Model file for the job. Use its own axes, mm. A direction names the side the tool comes from. Coordinates: 2 decimals unless noted, no trailing zeros. Loops run counter-clockwise (first coordinate to the right, second up) from the corner with the lowest first, then second, coordinate; pieces in that order, holes last.
from build123d import *

# Parameters (mm, degrees)
F0_W      = 47.7012
F0_H      = 9.5758
F1_DEPTH  = 7.8232
F2_R      = 2.3876
F3_DEPTH  = 9.53232
F2_R_2    = 3.0048968535
F2_R_3    = 2.9922132855
F2_R_4    = 2.9972531663
F4_DEPTH  = 0.762
F5_R      = 2.9885913722
F5_R_2    = 3.0048968535
F5_R_3    = 2.9922132855
F5_R_4    = 2.9972531663
F5_R_5    = 2.9570387739
F6_DEPTH  = 25.4
F7_R      = 3.0048968535
F7_R_2    = 2.3876
F7_R_3    = 2.9922132855
F7_R_4    = 2.9972531663
F7_R_5    = 2.9885913722
F7_R_6    = 2.9570387739
F8_DEPTH  = 0.762
F9_R      = 2.4384
F9_R_2    = 1.6002
F10_DEPTH = 0.9398
F11_W     = 45.9232
F11_H     = 6.0452
F12_DEPTH = 2.794


with BuildPart() as f1:
    # F0 (on Front) → F1 (new body)
    with BuildSketch(Plane.XZ):
        with Locations((-0.3360249102, 0.7659190055)):
            Rectangle(F0_W, F0_H)
    extrude(amount=F1_DEPTH)

    # F2 (on Front) → F3 (cut)
    with BuildSketch(Plane.XZ):
        with Locations((15.0480590754, 1.8556544835)):
            Circle(F2_R)
        with BuildLine():
            Line((5.7234941433, 0), (8.8326681668, 3.624302958))
            ThreePointArc((8.8326681668, 3.624302958), (5.4659296761, 3.3667384908), (5.7234941433, 0))
        make_face()
        with BuildLine():
            ThreePointArc((5.7234941433, 0), (8.275302748, -0.3572223603), (9.6656811551, 1.812151479))
            ThreePointArc((9.6656811551, 1.812151479), (9.4474549944, 2.8093730719), (8.8326681668, 3.624302958))
            Line((8.8326681668, 3.624302958), (5.7234941433, 0))
        make_face()
        with BuildLine():
            Line((-2.2399391754, 0.0756290061), (0.8692348481, 3.6999319641))
            ThreePointArc((0.8692348481, 3.6999319641), (-2.4975036427, 3.4423674968), (-2.2399391754, 0.0756290061))
        make_face()
        with BuildLine():
            ThreePointArc((-2.2399391754, 0.0756290061), (0.3118694292, -0.2815933542), (1.7022478363, 1.8877804851))
            ThreePointArc((1.7022478363, 1.8877804851), (1.4840216756, 2.885002078), (0.8692348481, 3.6999319641))
            Line((0.8692348481, 3.6999319641), (-2.2399391754, 0.0756290061))
        make_face()
        with BuildLine():
            Line((-9.9647576041, 0), (-7.3799977582, 4.0151651995))
            ThreePointArc((-7.3799977582, 4.0151651995), (-10.6799602808, 3.2999625227), (-9.9647576041, 0))
        make_face()
        with BuildLine():
            ThreePointArc((-9.9647576041, 0), (-7.5289295065, -0.0884040491), (-6.2847776811, 2.0075825997))
            ThreePointArc((-6.2847776811, 2.0075825997), (-6.5763910323, 3.1510307743), (-7.3799977582, 4.0151651995))
            Line((-7.3799977582, 4.0151651995), (-9.9647576041, 0))
        make_face()
        with BuildLine():
            Line((-17.9671654597, 0), (-15.2041278281, 3.8946319578))
            ThreePointArc((-15.2041278281, 3.8946319578), (-18.5329626228, 3.3288347947), (-17.9671654597, 0))
        make_face()
        with BuildLine():
            ThreePointArc((-17.9671654597, 0), (-15.4897179429, -0.1739039631), (-14.1980466439, 1.9473159789))
            ThreePointArc((-14.1980466439, 1.9473159789), (-14.4644267019, 3.0432446799), (-15.2041278281, 3.8946319578))
            Line((-15.2041278281, 3.8946319578), (-17.9671654597, 0))
        make_face()
    extrude(amount=F3_DEPTH, mode=Mode.SUBTRACT)

    # F2 (on Front) → F4 (cut)
    with BuildSketch(Plane.XZ):
        with BuildLine():
            ThreePointArc((-16.5209776811, 4.9036475293), (-16.5856466439, 4.9043547528), (-16.6503156067, 4.9036475293))
            Line((-16.6503156067, 4.9036475293), (-16.5209776811, 4.9036475293))
        make_face()
        with BuildLine():
            ThreePointArc((-5.6837863089, 2.0075825997), (-6.8384723861, 4.3673431298), (-9.41027084, 4.9036475293))
            ThreePointArc((-9.41027084, 4.9036475293), (-10.5062829761, -0.3521779303), (-5.6837863089, 2.0075825997))
        make_face()
        with BuildLine():
            ThreePointArc((-7.3799977582, 4.0151651995), (-6.5763910323, 3.1510307743), (-6.2847776811, 2.0075825997))
            ThreePointArc((-6.2847776811, 2.0075825997), (-7.5289295065, -0.0884040491), (-9.9647576041, 0))
            ThreePointArc((-9.9647576041, 0), (-10.6799602808, 3.2999625227), (-7.3799977582, 4.0151651995))
        make_face(mode=Mode.SUBTRACT)
        with BuildLine():
            Line((-16.5209776811, 4.9036475293), (-16.6503156067, 4.9036475293))
            ThreePointArc((-16.6503156067, 4.9036475293), (-18.5630084962, 4.1459788488), (-19.5185854293, 2.3240763694))
            ThreePointArc((-19.5185854293, 2.3240763694), (-18.8162584098, 0.0060665204), (-16.6174061088, -1.0095522371))
            ThreePointArc((-16.6174061088, -1.0095522371), (-14.5059634539, -0.1548248679), (-13.6286078699, 1.9473159789))
            ThreePointArc((-13.6286078699, 1.9473159789), (-14.4719642007, 4.0152678256), (-16.5209776811, 4.9036475293))
        make_face()
        with BuildLine():
            ThreePointArc((-15.2041278281, 3.8946319578), (-14.4644267019, 3.0432446799), (-14.1980466439, 1.9473159789))
            ThreePointArc((-14.1980466439, 1.9473159789), (-15.4897179429, -0.1739039631), (-17.9671654597, 0))
            ThreePointArc((-17.9671654597, 0), (-18.5329626228, 3.3288347947), (-15.2041278281, 3.8946319578))
        make_face(mode=Mode.SUBTRACT)
        with Locations((-0.6853521637, 1.8877804851)):
            Circle(F2_R_2)
        with BuildLine():
            ThreePointArc((0.8692348481, 3.6999319641), (1.4840216756, 2.885002078), (1.7022478363, 1.8877804851))
            ThreePointArc((1.7022478363, 1.8877804851), (0.3118694292, -0.2815933542), (-2.2399391754, 0.0756290061))
            ThreePointArc((-2.2399391754, 0.0756290061), (-2.4975036427, 3.4423674968), (0.8692348481, 3.6999319641))
        make_face(mode=Mode.SUBTRACT)
        with Locations((7.2780811551, 1.812151479)):
            Circle(F2_R_3)
        with BuildLine():
            ThreePointArc((8.8326681668, 3.624302958), (9.4474549944, 2.8093730719), (9.6656811551, 1.812151479))
            ThreePointArc((9.6656811551, 1.812151479), (8.275302748, -0.3572223603), (5.7234941433, 0))
            ThreePointArc((5.7234941433, 0), (5.4659296761, 3.3667384908), (8.8326681668, 3.624302958))
        make_face(mode=Mode.SUBTRACT)
        with Locations((15.0480590754, 1.8556544835)):
            Circle(F2_R_4)
        with Locations((15.0480590754, 1.8556544835)):
            Circle(F2_R, mode=Mode.SUBTRACT)
    extrude(amount=F4_DEPTH, mode=Mode.SUBTRACT)

    # F5 (on Front) → F6 (cut)
    with BuildSketch(Plane.XZ):
        with Locations((-8.6723776811, 2.0075825997)):
            Circle(F5_R)
        with Locations((-0.6853521637, 1.8877804851)):
            Circle(F5_R_2)
        with Locations((7.2780811551, 1.812151479)):
            Circle(F5_R_3)
        with Locations((15.0480590754, 1.8556544835)):
            Circle(F5_R_4)
        with Locations((-16.5856466439, 1.9473159789)):
            Circle(F5_R_5)
    extrude(amount=-F6_DEPTH, mode=Mode.SUBTRACT)

    # F7 (on face) → F8 (cut)
    with BuildSketch(Plane.XZ.offset(7.8232)):
        with Locations((-0.6853521637, 1.8877804851)):
            Circle(F7_R)
        with Locations((-0.6853521637, 1.8877804851)):
            Circle(F7_R_2, mode=Mode.SUBTRACT)
        with Locations((7.2780811551, 1.812151479)):
            Circle(F7_R_3)
        with Locations((7.2780811551, 1.812151479)):
            Circle(F7_R_2, mode=Mode.SUBTRACT)
        with Locations((15.0480590754, 1.8556544835)):
            Circle(F7_R_4)
        with Locations((15.0480590754, 1.8556544835)):
            Circle(F7_R_2, mode=Mode.SUBTRACT)
        with Locations((-8.6723776811, 2.0075825997)):
            Circle(F7_R_5)
        with Locations((-8.6723776811, 2.0075825997)):
            Circle(F7_R_2, mode=Mode.SUBTRACT)
        with Locations((-16.5856466439, 1.9473159789)):
            Circle(F7_R_6)
        with Locations((-16.5856466439, 1.9473159789)):
            Circle(F7_R_2, mode=Mode.SUBTRACT)
    extrude(amount=-F8_DEPTH, mode=Mode.SUBTRACT)

    # F9 (on face) → F10 (join)
    with BuildSketch(Plane.XY.offset(5.5538190055)):
        with Locations((-20.3004249102, -3.8862)):
            Circle(F9_R)
        with Locations((-20.3004249102, -3.8862)):
            Circle(F9_R_2, mode=Mode.SUBTRACT)
        with Locations((-12.1978249102, -3.8862)):
            Circle(F9_R)
        with Locations((-12.1978249102, -3.8862)):
            Circle(F9_R_2, mode=Mode.SUBTRACT)
        with Locations((-4.0952249102, -3.8862)):
            Circle(F9_R)
        with Locations((-4.0952249102, -3.8862)):
            Circle(F9_R_2, mode=Mode.SUBTRACT)
        with Locations((4.0952249102, -3.8862)):
            Circle(F9_R)
        with Locations((4.0952249102, -3.8862)):
            Circle(F9_R_2, mode=Mode.SUBTRACT)
        with Locations((12.1978249102, -3.8862)):
            Circle(F9_R)
        with Locations((12.1978249102, -3.8862)):
            Circle(F9_R_2, mode=Mode.SUBTRACT)
        with Locations((20.3004249102, -3.8862)):
            Circle(F9_R)
        with Locations((20.3004249102, -3.8862)):
            Circle(F9_R_2, mode=Mode.SUBTRACT)
    extrude(amount=F10_DEPTH)

    # F11 (on face) → F12 (cut)
    with BuildSketch(Plane(origin=(0, 0, -4.0219809945), x_dir=(1, 0, 0), z_dir=(0, 0, -1))):
        with Locations((-0.3360249102, 3.9116)):
            Rectangle(F11_W, F11_H)
    extrude(amount=-F12_DEPTH, mode=Mode.SUBTRACT)


solid = f1.part
Q1. Which spindle directions (+Z, -Z, +X, -X, +Y, -Y) get a long thin tool onto all of the face, cutting with end or side? Do faces 3 (the flat face through (-1, -4, 5.554)), 4 (the flat face through (-1, -4, -1.228)), 5 (the flat face through (-3, -0.762, 3)), 6 (the flat face through (22, -3, 6.494)), 7 (the flat face through (-0.7, 0, -1.3)). Say none if no direction does.
Answers:
face 3: +Z
face 4: -Z
face 5: +Y
face 6: +Z, +X, -X, +Y, -Y
face 7: +Z, -Z, +X, -X, +Y
Q2. Slice it at A-A (x = 0). List the corners of the cut face in (y, z), and give its area (3 significant figures).
Answers:
outline: (-7.82, -4.02) - (-6.93, -4.02) - (-6.93, -1.23) - (-0.89, -1.23) - (-0.89, -4.02) - (0, -4.02) - (0, -1.04) - (-0.76, -1.04) - (-0.76, -0.4) - (-7.06, -0.4) - (-7.06, -1.04) - (-7.82, -1.04) - close; (-7.82, 4.81) - (-7.06, 4.81) - (-7.06, 4.17) - (-0.76, 4.17) - (-0.76, 4.81) - (0, 4.81) - (0, 5.55) - (-7.82, 5.55) - close
area: 20.3 mm2
Q3. Drill centre lines: line 1 (X direction, y = -1.25, z = 1.25); line 2 (X direction, y = -7, z = 2.25); line 3 (Y direction, x = 6, z = -3.25). Where is each one in solid material? Low to high.
Answers:
line 1: x = -24.19 to -18.87, -14.3 to -10.94, -6.41 to -2.99, 1.62 to 4.96, 9.6 to 12.74, 17.36 to 23.51
line 2: x = -24.19 to -18.95, -14.22 to -11.05, -6.3 to -3.05, 1.67 to 4.93, 9.63 to 12.69, 17.4 to 23.51
line 3: y = -7.82 to -6.93, -0.89 to 0
Q4. Slice it at B-B (z = 1.25). Count the separate pieces of the cut face and the enclosed holes in it, and give its area (3 significant figures).
Answers:
separate pieces: 6
enclosed holes: 0
area: 184 mm2
Q5. Mould opens along X. For faces 1 (the flat face through (6, -4, 6.494)), 2 (the cylindrical face through (4.29, -7.45, 1.94)) say: +X half, -X half, draft (parallel to the pull), parting line (faces both ways), or undercut.
Answers:
face 1: draft
face 2: undercut
Q6. Flat gauge pins, fed straight in: P1, Ø3, axis at x = -8, z = 3, coming from the +Y side; P2, Ø1, axis at x = -9, y = -3.5, coming from the -Z side; P3, Ø1.6, axis at x = -12.5, y = -4, coming from the +Z side. Where does each tip first touch, or does it go through?
Answers:
P1: stops at y = -0.76
P2: stops at z = -1.23
P3: stops at z = 5.55
